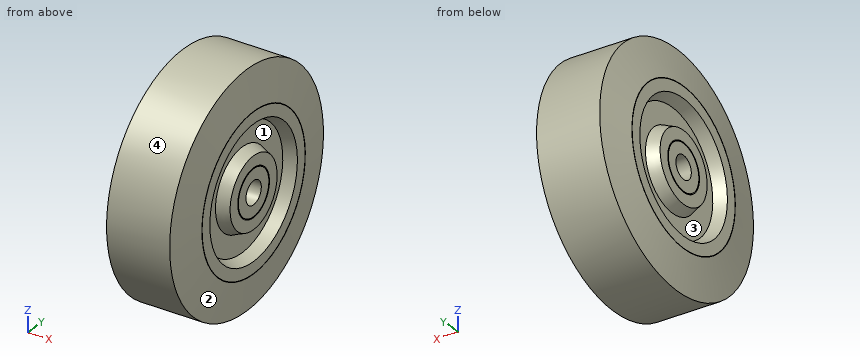
```python
from build123d import *

# Parameters (mm, degrees)
F2_R     = 47.0938119368
F3_DEPTH = 1


with BuildPart() as f1:
    # F0 (on Front) → F1 (revolve)
    with BuildSketch(Plane.XZ):
        Polygon((-20, -11.8900358561), (0, -11.8900358561), (20, -11.8900358561), (20, -6), (0, -6), (-20, -6), align=None)
    revolve(axis=Axis((-66.6633010662, 0, 0), (-1, 0, 0)))



with BuildPart() as f1b:
    # F0 (on Front) → F1, piece 2 (revolve)
    with BuildSketch(Plane.XZ):
        Polygon((-16.3393602265, -60), (0, -60), (16.3393602265, -60), (20, -40.3654314578), (0, -40.3654314578), (-20, -40.3654314578), align=None)
    revolve(axis=Axis((-66.6633010662, 0, 0), (-1, 0, 0)))


with BuildPart() as f1c:
    # F0 (on Front) → F1, piece 3 (revolve)
    with BuildSketch(Plane.XZ):
        Polygon((0, -40.1654314578), (20, -40.1654314578), (20, -34.172013402), (14.0782324597, -31.6885687669), (14.0782324597, -20.8386002505), (20, -18.3551556154), (20, -12.3617375596), (0, -12.3617375596), (-20, -12.3617375596), (-20, -18.3551556154), (-14.0782324597, -20.8386002505), (-14.0782324597, -31.6885687669), (-20, -34.172013402), (-20, -40.1654314578), align=None)
    revolve(axis=Axis((-66.6633010662, 0, 0), (-1, 0, 0)))


with BuildPart() as f1_1:
    add(f1.part)

    add(f1b.part)  # F3 merges F1b

    add(f1c.part)  # F3 merges F1c
    # F2 (on Right) → F3 (join, symmetric)
    with BuildSketch(Plane.YZ):
        Circle(F2_R)
    extrude(amount=F3_DEPTH, both=True)


solid = f1_1.part
```
Check sheet for the modelled part. Datum: model origin and axes. Units: mm. Face numbers are marked on the shaded views. A direction names the side the tool comes from. Give positions to 0.01 mm unless a question says otherwise; leave off trailing zeros. Write each loop counter-clockwise with the first axis right and the second up, starting at its lowest first coordinate (ties: lowest second). Pieces come first, ordered by that corner, then holes. Notation, with made-up numbers: (47.25, 65.25) -> (76.25, 65.25) arc R22 cw to (76.25, 74.25) -> close; hole circle Ø10 at (-36.5, 33). An arc over 180 degrees is marked (long way). Use CSV: the item, a comma, the result in double quotes. Start each with the question number.
Q1. Scan lines: line 1 along Y through (x, z) = (9.5, 0); line 2 along Y through (x, z) = (-10, 2.5). Record each from-to range of solid material in increasing order.
Q2. Release check for a two-part mould opening along Z. For the marked faces 1 and 2 record: +Z half, -Z half, draft (parallel to the pull), parting line (faces both ways), or undercut.
Q3. Tool access check on the marked faces 3 and 4. Record the directions out of +Z, -Z, +X, -X, +Y, -Y that give a thin tool (end or side, any length) a straight path to the whole face; none if there is none.
Q4. Cross-section at A-A on x = -7.5. Enter the section's corners in (y, z), and give its area (3 significant figures).
Q5. Depth check by flat-ended pin: P1, Ø3, axis at y = 23, z = -2.5, coming from the -X side; P2, Ø6, axis at y = -2.5, z = 1, coming from the +X side; P3, Ø10, axis at x = -2.5, z = -34.5, coming from the -Y side. Enter the tip coordinate at first touch or a pass-through.
Working result:
1,line 1,"y = -60 to -40.37, -40.17 to -12.36, -11.89 to -6, 6 to 11.89, 12.36 to 40.17, 40.37 to 60"
1,line 2,"y = -59.95 to -40.29, -40.09 to -12.11, -11.62 to -5.45, 5.45 to 11.62, 12.11 to 40.09, 40.29 to 59.95"
2,face 1,"undercut"
2,face 2,"parting line"
3,face 3,"-X"
3,face 4,"+X, -X"
4,outline,"circle Ø120 at (0, 0); circle Ø80.33 at (0, 0); circle Ø23.78 at (0, 0); hole circle Ø80.73 at (0, 0); hole circle Ø24.72 at (0, 0); hole circle Ø12 at (0, 0)"
4,area,"11,100 mm^2"
5,P1,"stops at x = -14.08"
5,P2,"stops at x = 1"
5,P3,"stops at y = -52.25"
